Solid Edge part; units mm, degrees
sketch "Sketch1" plane through (0, 0, 0) normal (0, -1, 0) x (1, 0, 0)
  line L0 (60, 53) -> (0, 53)
  line L1 (0, 0) -> (0, 53)
  line L2 (0, 0) -> (-30, 0)
  line L3 (-30, 0) -> (-30, -12)
  line L4 (-30, -12) -> (12, -12)
  line L5 (12, -12) -> (12, 41)
  line L6 (12, 41) -> (48, 41)
  line L7 (48, 41) -> (48, -12)
  line L8 (48, -12) -> (90, -12)
  line L9 (90, -12) -> (90, 0)
  line L10 (90, 0) -> (60, 0)
  line L11 (60, 0) -> (60, 53)
extrude "Protrusion1" add sketch "Sketch1" against normal blind 40
sketch "Sketch2" plane through (30, 20, 53) normal (0, 0, 1) x (1, 0, 0)
  circle A0 centre (-45, 0) radius 6
  circle A1 centre (45, 0) radius 6
  circle A2 centre (0, 0) radius 12.5
extrude "ExtrudedCutout_1" cut sketch "Sketch2" against normal blind 65
Can you work these out from the model? Positions are in its coordinate system, mm. A direction names the side the tool comes from. Round coordinates to 2 decimals unless told otherwise and drop trailing zeros. Loops run counter-clockwise (first coordinate to the right, second up) from the corner with the lowest first, then second, coordinate; pieces in that order, holes last. Notation, with made-up numbers: (63.5, 6) -> (89.5, 6) arc R25 cw to (89.5, 27) -> close; hole circle Ø10 at (24.5, -4.5). An arc over 180 degrees is marked (long way). Answer in a Markdown table with one row per item.
Item 1: We'd pull the mould along X, two halves only. Please class faces 1 (the cylindrical face through (69, 20, -6)), 2 (the flat face through (82, 20, 0)), 3 (the flat face through (-30, 20, -6)): released by +X, released by -X, zero draft, split by the parting line, or undercut.
Answer block:
| item | result |
|---|---|
| face 1 | undercut |
| face 2 | zero draft |
| face 3 | released by -X |
Item 2: On a 3-axis mill with a long thin cutter (end or side, diameter ignored), from which of +Z, -Z, +X, -X, +Y, -Y can I reach the whole of each face in a straight line? I mean faces 4 (the cylindrical face through (20.08, 12.394, 47.084)), 5 (the flat face through (90, 20, -6)), 6 (the flat face through (-8, 20, 0)), 7 (the flat face through (12, 20, 14)), 8 (the flat face through (60, 20, 26)). Say none if no direction works.
Answer block:
| item | result |
|---|---|
| face 4 | +Z, -Z |
| face 5 | +Z, -Z, +X, +Y, -Y |
| face 6 | +Z, -X, +Y, -Y |
| face 7 | -Z, +Y, -Y |
| face 8 | +Z, +X, +Y, -Y |
Item 3: Will these pins go through, and if not, where does the flat tip stop? P1, Ø20, axis at y = 27.5, z = 37.5, coming from the -X side; P2, Ø6, axis at y = 24, z = 14.5, coming from the +X side; P3, Ø9, axis at x = -19.5, y = 16.5, coming from the +Z side.
Answer block:
| item | result |
|---|---|
| P1 | x = 0 |
| P2 | x = 60 |
| P3 | z = 0 |
Item 4: Suppose I cut it at A-A, the plane x = -15. List the corners of the cut face in (y, z) for me, plus the area to 3 significant figures.
Answer block:
| item | result |
|---|---|
| outline | (0, -12) -> (14, -12) -> (14, 0) -> (0, 0) -> close; (26, -12) -> (40, -12) -> (40, 0) -> (26, 0) -> close |
| area | 336 mm² |
Item 5: Suppose I cut it at D-D, the plane y = 36. List the corners of the cut face in (x, z) for me.
Answer block:
| item | result |
|---|---|
| outline | (-30, -12) -> (12, -12) -> (12, 41) -> (48, 41) -> (48, -12) -> (90, -12) -> (90, 0) -> (60, 0) -> (60, 53) -> (0, 53) -> (0, 0) -> (-30, 0) -> close |
Item 6: Suppose I cut it at C-C, the plane z = 11.5. List the corners of the cut face in (x, y) for me, plus the area to 3 significant figures.
Answer block:
| item | result |
|---|---|
| outline | (0, 0) -> (12, 0) -> (12, 40) -> (0, 40) -> close; (48, 0) -> (60, 0) -> (60, 40) -> (48, 40) -> close |
| area | 960 mm² |
Item 7: Suppose I cut it at B-B, the plane y = 20. List the corners of the cut face in (x, z) for me.
Answer block:
| item | result |
|---|---|
| outline | (-30, -12) -> (-21, -12) -> (-21, 0) -> (-30, 0) -> close; (-9, -12) -> (12, -12) -> (12, 41) -> (17.5, 41) -> (17.5, 53) -> (0, 53) -> (0, 0) -> (-9, 0) -> close; (42.5, 41) -> (48, 41) -> (48, -12) -> (69, -12) -> (69, 0) -> (60, 0) -> (60, 53) -> (42.5, 53) -> close; (81, -12) -> (90, -12) -> (90, 0) -> (81, 0) -> close |
Item 8: If I drill on probe 1 along X at (y, z) = (18, 28); probe 2 along Y at (x, z) = (30, 46); probe 3 along Y at (x, z) = (-15, -6), over which ranges is the centre line in solid material (lowest first)?
Answer block:
| item | result |
|---|---|
| probe 1 | 0 to 12, 48 to 60 |
| probe 2 | 0 to 7.5, 32.5 to 40 |
| probe 3 | 0 to 14, 26 to 40 |
